```python
from build123d import *

# Parameters (mm, degrees)
GENERALSHAPE_DEPTH   = 0.8
ADDTOLERANCE_START   = -0.8
ADDTOLERANCE_DEPTH   = 1.6
BACKPLANE_DEPTH      = 71.573791169
BACKPLANE_DEPTH_BACK = 71.573791169
FILLET2_R            = 0.8636


# Read off the part's stored shape, not the designer's step: AddTolerance
with BuildPart() as part:
    # Sketch2 → GeneralShape (new, symmetric)
    with BuildSketch(Plane(origin=(0, 0, 0), x_dir=(1, 0, 0), z_dir=(0, 1, 0))):
        Polygon((47.4, 46.4), (37, 46.4), (37, 50), (-37, 50), (-37, 46.4), (-47.4, 46.4), (-47.4, 41.5), (-50, 41.5), (-50, -38.9), (-41.5, -47.4), (41.5, -47.4), (50, -38.9), (50, 41.5), (47.4, 41.5), align=None)
    extrude(amount=GENERALSHAPE_DEPTH, both=True)

    # AddTolerance outline → AddTolerance (cut)
    with BuildSketch(Plane(origin=(0, 0, 0), x_dir=(1, 0, 0), z_dir=(0, 1, 0)).offset(ADDTOLERANCE_START)):
        Polygon((49.9, 41.4), (49.9, -39), (50, -38.9), (50, 41.5), (47.4, 41.5), (47.4, 46.4), (37, 46.4), (37, 50), (-37, 50), (-37, 46.4), (-47.4, 46.4), (-47.4, 41.5), (-50, 41.5), (-50, -38.9), (-49.9, -39), (-49.9, 41.4), (-47.3, 41.4), (-47.3, 46.3), (-36.9, 46.3), (-36.9, 49.9), (36.9, 49.9), (36.9, 46.3), (47.3, 46.3), (47.3, 41.4), align=None)
    extrude(amount=ADDTOLERANCE_DEPTH, mode=Mode.SUBTRACT)

    # Sketch4 → Backplane (cut, two sides: drawn at the far end of the back side and taken through both)
    with BuildSketch(Plane(origin=(0, 0, 0), x_dir=(1, 0, 0), z_dir=(0, 1, 0)).offset(-BACKPLANE_DEPTH_BACK)):
        with BuildLine():
            Line((41.5, -47.4), (44.1, -44.8))
            Line((44.1, -44.8), (41.232050808, -44.8))
            ThreePointArc((41.232050808, -44.8), (39.5, -43.8), (37.767949192, -44.8))
            Line((37.767949192, -44.8), (18.232050808, -44.8))
            ThreePointArc((18.232050808, -44.8), (16.5, -43.8), (14.767949192, -44.8))
            Line((14.767949192, -44.8), (-14.767949192, -44.8))
            ThreePointArc((-14.767949192, -44.8), (-16.5, -43.8), (-18.232050808, -44.8))
            Line((-18.232050808, -44.8), (-37.767949192, -44.8))
            ThreePointArc((-37.767949192, -44.8), (-39.5, -43.8), (-41.232050808, -44.8))
            Line((-41.232050808, -44.8), (-44.1, -44.8))
            Line((-44.1, -44.8), (-41.5, -47.4))
            Line((-41.5, -47.4), (41.5, -47.4))
        make_face()
    extrude(amount=BACKPLANE_DEPTH + BACKPLANE_DEPTH_BACK, mode=Mode.SUBTRACT)

    # Fillet2
    fillet2_edges = [part.edges().sort_by_distance(p)[0] for p in [
        (47.3, 0, -41.4),
        (36.9, 0, -46.3),
        (-36.9, 0, -46.3),
        (-47.3, 0, -41.4),
    ]]
    fillet(fillet2_edges, radius=FILLET2_R)


solid = part.part
```
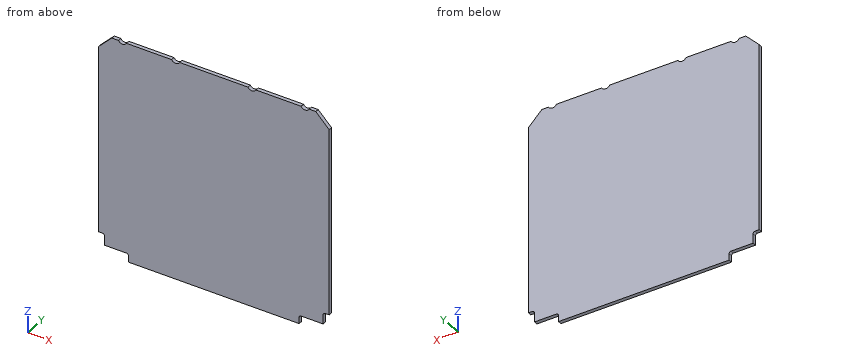
The listing builds one solid part. Answer for the finished solid, in the listing's coordinates (mm). Coordinates: 2 decimals unless noted, no trailing zeros. Write each loop counter-clockwise with the first axis right and the second up, starting at its lowest first coordinate (ties: lowest second). Pieces come first, ordered by that corner, then holes. Notation, with made-up numbers: M 2,34 L 50,34 A9 cw 50,43 Z; hole C -34.5,-14.75 d4. An arc over 180 degrees is marked long. Use a Markdown table: item, result. Add a question column.
1. Given P1, Ø0.8, axis at x = 40.5, y = 0, coming from the -Z side; P2, Ø0.5, axis at y = -0.5, z = -45, coming from the -X side; P3, Ø0.5, axis at y = 0, z = -49, coming from the +X side, each flat-ended and moving along its own axis, determine where each tip first touches the part or whether it passes through.
2. Section A-A (y = 0.5) is taken. Give the vertices of the cut face in (x, z).
3. Straight lines are drawn through the part: line 1 along Z through (x, y) = (45.5, -0.3); line 2 along Z through (x, y) = (40.5, -0.3). For each, find the intervals that lie inside material, in ascending order. Write a range as [from, to].
Data:
| question | item | result |
|---|---|---|
| 1 | P1 | stops at z = -46.3 |
| 1 | P2 | stops at x = -47.3 |
| 1 | P3 | stops at x = 36.9 |
| 2 | outline | M -49.9,-41.4 L -48.16,-41.4 A0.86 cw -47.3,-42.26 L -47.3,-46.3 L -37.76,-46.3 A0.86 cw -36.9,-47.16 L -36.9,-49.9 L 36.9,-49.9 L 36.9,-47.16 A0.86 cw 37.76,-46.3 L 47.3,-46.3 L 47.3,-42.26 A0.86 cw 48.16,-41.4 L 49.9,-41.4 L 49.9,39 L 44.1,44.8 L 41.23,44.8 A2 cw 37.77,44.8 L 18.23,44.8 A2 cw 14.77,44.8 L -14.77,44.8 A2 cw -18.23,44.8 L -37.77,44.8 A2 cw -41.23,44.8 L -44.1,44.8 L -49.9,39 Z |
| 3 | line 1 | z = [-46.3, 43.4] |
| 3 | line 2 | z = [-46.3, 44.07] |
